Drawing for the job (mm, zero at the part's lowest x, y, z). A direction names the side the tool comes from. Give positions to 0.01 mm unless a question says otherwise; leave off trailing zeros. Order: outer loops, then holes, each group sorted by start corner. A loop starts at its lowest first (then second) coordinate and runs counter-clockwise, first axis right, second up. Notation, with made-up numbers: M -3,56.25 L 5,56.25 A19 ccw 5,81.25 Z; hole C 42,-32 d11. An arc over 180 degrees is marked long. One line per item, written item: value.
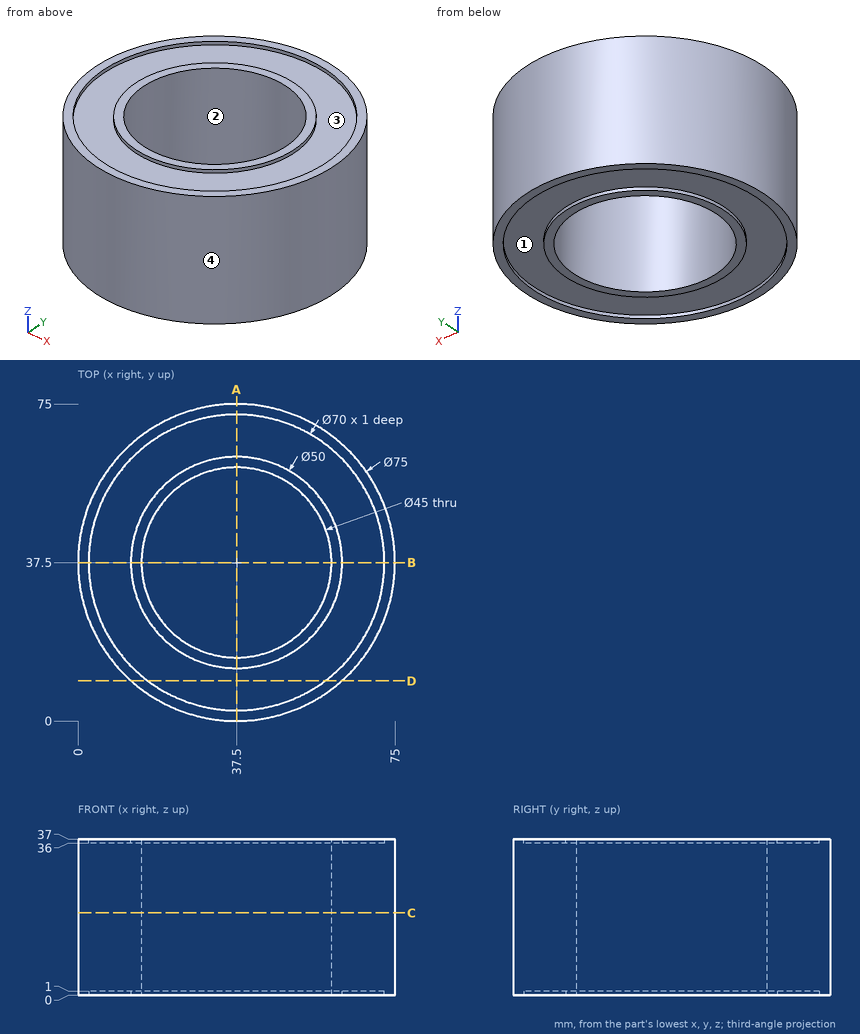
1) Saw through at C-C, the plane z = 19.5. Write the cut outline in (x, y), then the cut area to 3 significant figures.
Check values:
outline: C 37.5,37.5 d75; hole C 37.5,37.5 d45
area: 2,830 mm^2
2) Saw through at A-A, the plane x = 37.5. Write the cut outline in (y, z).
Check values:
outline: M 0,0 L 2.5,0 L 2.5,1 L 12.5,1 L 12.5,0 L 15,0 L 15,37 L 12.5,37 L 12.5,36 L 2.5,36 L 2.5,37 L 0,37 Z; M 60,0 L 62.5,0 L 62.5,1 L 72.5,1 L 72.5,0 L 75,0 L 75,37 L 72.5,37 L 72.5,36 L 62.5,36 L 62.5,37 L 60,37 Z
3) Pin check, flat tips, straight feed: pin 1 (5 mm diameter, centred on y = 63.5, z = 21, fed in from +X); pin 2 (1.5 mm diameter, centred on x = 14, z = 17.5, fed in from -Y); pin 3 (6 mm diameter, centred on y = 44, z = 31.5, fed in from -X); pin 4 (1.5 mm diameter, centred on x = 23, y = 23.5, fed in from +Z). Stop position of each tip, or through.
Check values:
pin 1: x = 66.72
pin 2: y = 7.69
pin 3: x = 0.16
pin 4: through
4) Tool access for the marked faces 1 and 2: list every direction of +Z, -Z, +X, -X, +Y, -Y with a clear straight run to the whole face (end or side of a thin tool).
Check values:
face 1: -Z
face 2: +Z, -Z
5) Saw through at D-D, the plane y = 9.5. Write the cut outline in (x, z).
Check values:
outline: M 12.56,0 L 16.5,0 L 16.5,1 L 58.5,1 L 58.5,0 L 62.44,0 L 62.44,37 L 58.5,37 L 58.5,36 L 16.5,36 L 16.5,37 L 12.56,37 Z
6) Mould opens along Y. For the marked faces 3 and 4 say: released by +Y, released by -Y, zero draft, split by the parting line, or undercut.
Check values:
face 3: undercut
face 4: split by the parting line
7) Drill centre lines: probe 1 along Y at (x, z) = (37.5, 0.85); probe 2 along Z at (x, y) = (52, 61); probe 3 along X at (y, z) = (28, 25.5). Where is each one in solid material? Low to high. Write a range as from..to.
Check values:
probe 1: 0..2.5, 12.5..15, 60..62.5, 72.5..75
probe 2: 1..36
probe 3: 1.22..17.1, 57.9..73.78
